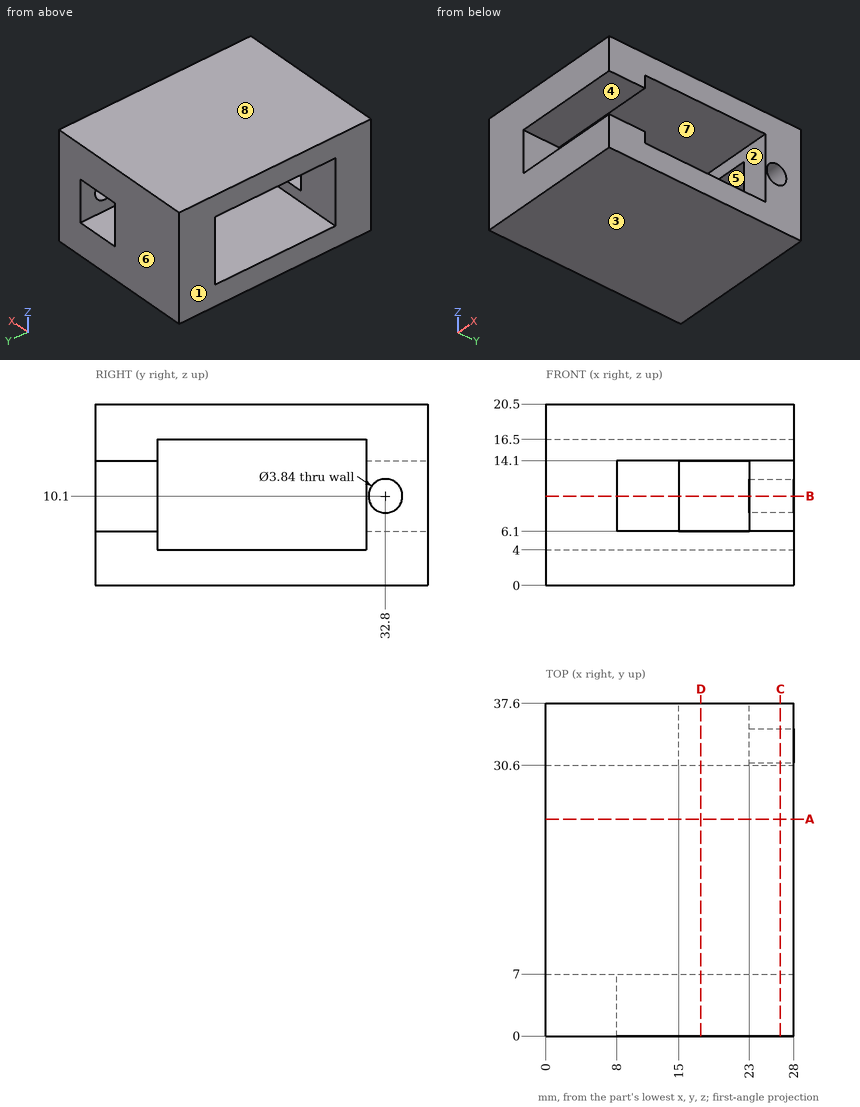
Source: three-view drawing plus pictorial views. Frame: mm from the lowest corner of the part. A direction names the side the tool comes from. Give positions to 0.01 mm unless a question says otherwise; leave off trailing zeros. Loops run counter-clockwise (first coordinate to the right, second up) from the corner with the lowest first, then second, coordinate; pieces in that order, holes last. Notation, with made-up numbers: M 48.5,48.5 L 70.5,48.5 A17 cw 70.5,69.5 Z; hole C 63.25,86.25 d6. An arc over 180 degrees is marked long. Use CSV: the item, a comma, the result in double quotes.
(1) Set-up query: the marked faces 4, 5, 6, 7 and 8. Return all of +Z, -Z, +X, -X, +Y, -Y with unobstructed straight access to the full face (end or side cutting, diameter ignored); none if empty.
Outcome:
face 4,"+X, -Y"
face 5,"+Y, -Y"
face 6,"+Z, -Z, +X, -X, +Y"
face 7,"+X, -X"
face 8,"+Z, +X, -X, +Y, -Y"
(2) Pull-direction query (Z, two-part tool) for the marked faces 1, 2 and 3; classes: pulls with the +Z half, pulls with the -Z half, needs draft (parallel to the pull), parting line crosses it, or undercut.
Outcome:
face 1,"needs draft"
face 2,"undercut"
face 3,"pulls with the -Z half"
(3) Material intervals for L1, parallel to Z at x = 11.75, y = 8.5; L2, parallel to Y at x = 24.6, z = 10.1; L3, parallel to Z at x = 21.25, y = 6, sorted ascending. Write a range as [from, to].
Outcome:
L1,"z = [0, 4], [16.5, 20.5]"
L2,"y = [30.6, 30.88], [34.72, 37.6]"
L3,"z = [0, 6.1], [14.1, 20.5]"
(4) Section D-D, the plane x = 17.5. Return loops of the section in (y, z).
Outcome:
outline,"M 0,0 L 37.6,0 L 37.6,6.1 L 30.6,6.1 L 30.6,4 L 7,4 L 7,6.1 L 0,6.1 Z; M 0,14.1 L 7,14.1 L 7,16.5 L 30.6,16.5 L 30.6,14.1 L 37.6,14.1 L 37.6,20.5 L 0,20.5 Z"
(5) Section C-C, the plane x = 26.5. Return loops of the section in (y, z), plus the area to 3 significant figures.
Outcome:
outline,"M 0,0 L 37.6,0 L 37.6,20.5 L 0,20.5 L 0,14.1 L 7,14.1 L 7,16.5 L 30.6,16.5 L 30.6,4 L 7,4 L 7,6.1 L 0,6.1 Z; hole C 32.8,10.1 d3.84"
area,"408 mm²"
(6) Pin query (flat end, axial travel): P1, Ø7.5, axis at y = 2.5, z = 10, coming from the +X side; P2, Ø1, axis at y = 9, z = 8.5, coming from the +X side. Return the tip coordinate at first contact, or that it passes through.
Outcome:
P1,"stops at x = 8"
P2,"passes through"
(7) Section A-A, the plane y = 24.5. Return loops of the section in (x, z).
Outcome:
outline,"M 0,0 L 28,0 L 28,4 L 0,4 Z; M 0,16.5 L 28,16.5 L 28,20.5 L 0,20.5 Z"
(8) Section B-B, the plane z = 10.1. Return loops of the section in (x, y).
Outcome:
outline,"M 0,0 L 8,0 L 8,7 L 0,7 Z; M 0,30.6 L 15,30.6 L 15,37.6 L 0,37.6 Z; M 23,30.6 L 28,30.6 L 28,30.88 L 23,30.88 Z; M 23,34.72 L 28,34.72 L 28,37.6 L 23,37.6 Z"
